Read the model definition and answer for the solid it produces. Units are mm, in the model's axes. Face numbers are marked on the shaded views. Coordinates: 2 decimals unless noted, no trailing zeros. Loops run counter-clockwise (first coordinate to the right, second up) from the corner with the lowest first, then second, coordinate; pieces in that order, holes last.
Q1. Straight lines are drawn through the part: line 1 (X direction, y = 41.5, z = 0); line 2 (X direction, y = 23.5, z = 0); line 3 (Z direction, x = -7.5, y = 4). For each, find the intervals that lie inside material, in ascending order.
Q2. Section C-C (x = 0) is taken. Give the vertices of the cut face in (y, z).
Q3. The mould has two halves that part along X. Classify the marked faces 1, 2, 3 and 4: pulls with the +X half, pulls with the -X half, needs draft (parallel to the pull), parting line crosses it, or undercut.
Q4. Flat-ended cylindrical pins translate along their axes: P1, Ø2, axis at x = -10.5, z = 5, coming from the +Y side; P2, Ø2, axis at x = 12.22, z = -4.45, coming from the +Y side; P3, Ø5, axis at x = 12.22, z = -4.45, coming from the -Y side; P4, Ø6, axis at x = -11.5, y = 39, coming from the +Z side. Find the tip coordinate at first contact, or state that the pin passes through.
Q5. Section D-D (y = 39.5) is taken. Give the vertices of the cut face in (x, z), then the cut area to 3 significant figures.
Q6. Section A-A (z = 0) is taken. Give the vertices of the cut face in (x, y), then the cut area to 3 significant figures.
Q7. Section B-B (y = 31.5) is taken. Give the vertices of the cut face in (x, z), then the cut area to 3 significant figures.
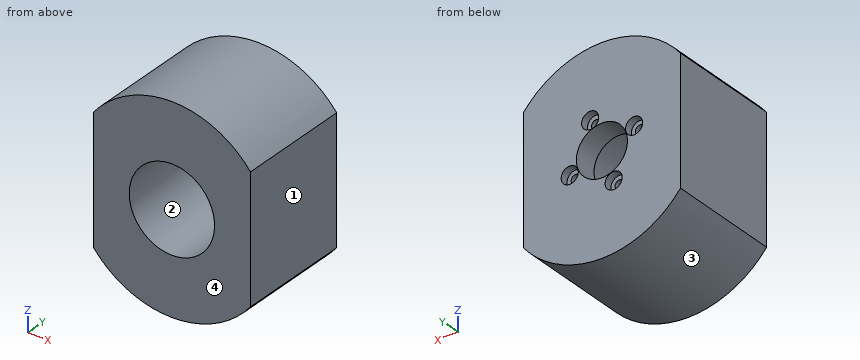
from build123d import *

# Parameters (mm, degrees)
BOSS_EXTRUDE1_DEPTH            = 44
CBORE_FOR_M3_SHCS1_D           = 3.4
CBORE_FOR_M3_SHCS1_CBORE_D     = 6.5
CBORE_FOR_M3_SHCS1_CBORE_DEPTH = 3
CIRPATTERN1_COUNT              = 4
SKETCH4_R                      = 16.2
CUT_EXTRUDE1_DEPTH             = 35
SKETCH5_R                      = 9.7
CUT_EXTRUDE2_DEPTH             = 66.498740446


with BuildPart() as part:
    # Sketch1 → Boss-Extrude1 (new body)
    with BuildSketch(Plane(origin=(0, 0, 0), x_dir=(1, 0, 0), z_dir=(0, 1, 0))):
        with BuildLine():
            Line((-29.85, 23.917357714), (-29.85, -23.917357714))
            ThreePointArc((-29.85, -23.917357714), (0, -38.25), (29.85, -23.917357714))
            Line((29.85, -23.917357714), (29.85, 23.917357714))
            ThreePointArc((29.85, 23.917357714), (0, 38.25), (-29.85, 23.917357714))
        make_face()
    extrude(amount=BOSS_EXTRUDE1_DEPTH)

    # CBORE for M3 SHCS1 (through all)
    with Locations(Plane(origin=(0, 44, 0), x_dir=(1, 0, 0), z_dir=(0, 1, 0))):
        with Locations((-4.446261863, 12.21600407)):
            cbore_for_m3_shcs1 = CounterBoreHole(CBORE_FOR_M3_SHCS1_D / 2, CBORE_FOR_M3_SHCS1_CBORE_D / 2, CBORE_FOR_M3_SHCS1_CBORE_DEPTH)

    # CirPattern1: CBORE for M3 SHCS1 ×4 about axis
    cirpattern1_axis = Axis((0, 0, 0), (0, 1, 0))
    for i in range(1, CIRPATTERN1_COUNT):
        add(cbore_for_m3_shcs1.rotate(cirpattern1_axis, i * 360 / CIRPATTERN1_COUNT), mode=Mode.SUBTRACT)

    # Sketch4 → Cut-Extrude1 (cut)
    with BuildSketch(Plane.XZ):
        with Locations(Location((0, 0, 0), (0, 0, 270))):
            Circle(SKETCH4_R)
    extrude(amount=-CUT_EXTRUDE1_DEPTH, mode=Mode.SUBTRACT)

    # Sketch5 → Cut-Extrude2 (cut, through all)
    with BuildSketch(Plane(origin=(0, 44, 0), x_dir=(1, 0, 0), z_dir=(0, 1, 0))):
        with Locations(Location((0, 0, 0), (0, 0, 270))):
            Circle(SKETCH5_R)
    extrude(amount=-CUT_EXTRUDE2_DEPTH, mode=Mode.SUBTRACT)


solid = part.part
Numbers:
1. line 1: x = -29.85 to -9.7, 9.7 to 29.85
1. line 2: x = -29.85 to -16.2, 16.2 to 29.85
1. line 3: z = -37.51 to -14.36, 14.36 to 37.51
2. outline: (0, -38.25) - (44, -38.25) - (44, -9.7) - (35, -9.7) - (35, -16.2) - (0, -16.2) - close; (0, 16.2) - (35, 16.2) - (35, 9.7) - (44, 9.7) - (44, 38.25) - (0, 38.25) - close
3. face 1: pulls with the +X half
3. face 2: undercut
3. face 3: parting line crosses it
3. face 4: needs draft
4. P1: stops at y = 41
4. P2: passes through
4. P3: stops at y = 35
4. P4: stops at z = 37.29
5. outline: (-29.85, -23.92) arc R38.25 ccw to (29.85, -23.92) - (29.85, 23.92) arc R38.25 ccw to (-29.85, 23.92) - close; hole circle Ø3.4 at (-12.22, 4.45); hole circle Ø19.4 at (0, 0); hole circle Ø3.4 at (-4.45, -12.22); hole circle Ø3.4 at (4.45, 12.22); hole circle Ø3.4 at (12.22, -4.45)
5. area: 3,720 mm2
6. outline: (-29.85, 0) - (-16.2, 0) - (-16.2, 35) - (-9.7, 35) - (-9.7, 44) - (-29.85, 44) - close; (9.7, 35) - (16.2, 35) - (16.2, 0) - (29.85, 0) - (29.85, 44) - (9.7, 44) - close
6. area: 1,320 mm2
7. outline: (-29.85, -23.92) arc R38.25 ccw to (29.85, -23.92) - (29.85, 23.92) arc R38.25 ccw to (-29.85, 23.92) - close; hole circle Ø32.4 at (0, 0)
7. area: 3,220 mm2
